Autodesk Inventor part; units mm, degrees
ref_plane "YZ Plane" through (0, 0, 0) normal (1, 0, 0) x (0, 1, 0)
ref_plane "XZ Plane" through (0, 0, 0) normal (0, 1, 0) x (-1, 0, 0)
ref_plane "XY Plane" through (0, 0, 0) normal (0, 0, 1) x (1, 0, 0)
sketch "Sketch1" plane through (0, 0, 0) normal (0, 0, 1) x (1, 0, 0)
  line L0 (-12.7, -12.7) -> (12.7, -12.7)
  line L1 (12.7, -12.7) -> (12.7, 12.7)
  line L2 (12.7, 12.7) -> (-12.7, 12.7)
  line L3 (-12.7, 12.7) -> (-12.7, -12.7)
  line L4 (-12.7, -12.7) -> (12.7, 12.7) construction
  line L5 (12.7, -12.7) -> (-12.7, 12.7) construction
  line L6 (11.1125, -11.1125) -> (-11.1125, -11.1125)
  line L7 (-11.1125, -11.1125) -> (-11.1125, 11.1125)
  line L8 (-11.1125, 11.1125) -> (11.1125, 11.1125)
  line L9 (11.1125, 11.1125) -> (11.1125, -11.1125)
  line L10 (11.1125, -11.1125) -> (-11.1125, 11.1125) construction
  line L11 (-11.1125, -11.1125) -> (11.1125, 11.1125) construction
  point P0 (0, 0)
  dimension "d0" = 25.4
  dimension "d1" = 25.4
  dimension "d3" = 22.225
  dimension "d4" = 22.225
extrude "Extrusion1" add sketch "Sketch1" along normal mid plane 101.6
sketch "Sketch2" plane through (-12.7, 12.7, 50.8) normal (0, 1, 0) x (1, 0, 0)
  line L0 (25.4, 0) -> (0, 0)
  point P0 (12.7, 50.8)
  point P1 (12.7, 6.35)
  point P2 (12.7, 31.75)
  point P3 (12.7, 57.15)
  point P4 (12.7, 0)
  point P5 (12.7, 0)
  dimension "d7" = 6.35
  dimension "d8" = 25.4
  dimension "d9" = 25.4
hole "Hole1" at (0, 12.7, 44.45) at (0, 12.7, 19.05) at (0, 12.7, -6.35) direction (0, -1, 0) diameter 5.1054 end through all
properties part number "DB1-012" material "Aluminum 6061"
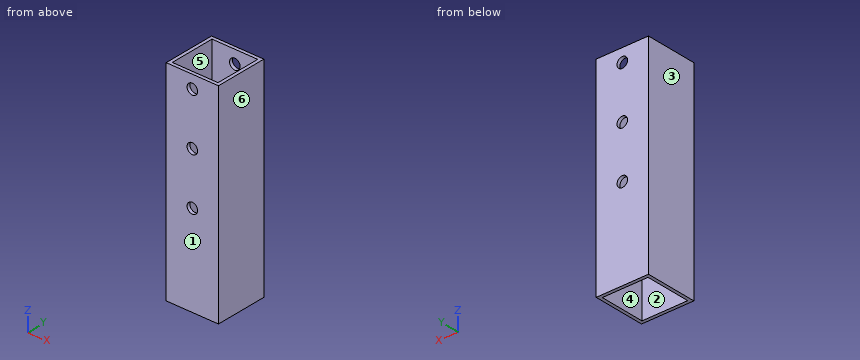
Check sheet for the modelled part. Datum: model origin and axes. Units: mm. Face numbers are marked on the shaded views. A direction names the side the tool comes from. Give positions to 0.01 mm unless a question says otherwise; leave off trailing zeros. Order: outer loops, then holes, each group sorted by start corner. A loop starts at its lowest first (then second) coordinate and runs counter-clockwise, first axis right, second up. Notation, with made-up numbers: (64.5, 35) -> (98.5, 35) arc R14 ccw to (98.5, 45) -> close; hole circle Ø9 at (-30.5, 22). An arc over 180 degrees is marked (long way). Use CSV: the item, a comma, the result in double quotes. Start each with the question number.
1) Set-up check for the marked faces 5 and 6: record each of +Z, -Z, +X, -X, +Y, -Y from which the full face is reachable in a straight line by a thin tool's end or side.
2) Sectioned sample at D-D, the plane x = 0. Give the number of separate pieces and of enclosed holes in the cut face, plus the area to 3 significant figures.
3) Sectioned sample at A-A, the plane z = 19.05. Record the boundary of the cut face in (x, y), plus the area to 3 significant figures.
4) Go/stop test with a flat-tipped pin: P1, Ø3, axis at x = 0, z = -6.35, coming from the -Y side. Record where the tip stops, or that it passes through.
5) Mould release check, pull along X, two halves, no side actions. Record for the marked faces 1, 2, 3 and 4: released by +X, released by -X, zero draft, split by the parting line, or undercut.
6) Material ranges on line 1 (Z direction, x = 0, y = 12.4); line 2 (X direction, y = -12.2, z = 44.45); line 3 (Y direction, x = -10, z = 32), recorded low to high. Write a range as from..to.
7) Sectioned sample at B-B, the plane x = 7.75. Record the boundary of the cut face in (y, z).
Recorded:
1,face 5,"+Z, -Z"
1,face 6,"+Z, -Z, +X, +Y, -Y"
2,separate pieces,"8"
2,enclosed holes,"0"
2,area,"274 mm2"
3,outline,"(-12.7, -12.7) -> (-2.55, -12.7) -> (-2.55, -11.11) -> (-11.11, -11.11) -> (-11.11, 11.11) -> (-2.55, 11.11) -> (-2.55, 12.7) -> (-12.7, 12.7) -> close; (2.55, -12.7) -> (12.7, -12.7) -> (12.7, 12.7) -> (2.55, 12.7) -> (2.55, 11.11) -> (11.11, 11.11) -> (11.11, -11.11) -> (2.55, -11.11) -> close"
3,area,"135 mm2"
4,P1,"through"
5,face 1,"zero draft"
5,face 2,"undercut"
5,face 3,"released by -X"
5,face 4,"undercut"
6,line 1,"-50.8..-8.9, -3.8..16.5, 21.6..41.9, 47..50.8"
6,line 2,"-12.7..-2.55, 2.55..12.7"
6,line 3,"-12.7..-11.11, 11.11..12.7"
7,outline,"(-12.7, -50.8) -> (-11.11, -50.8) -> (-11.11, 50.8) -> (-12.7, 50.8) -> close; (11.11, -50.8) -> (12.7, -50.8) -> (12.7, 50.8) -> (11.11, 50.8) -> close"
